from build123d import *

# Parameters (mm, degrees)
SKETCH_W             = 185.32
SKETCH_H             = 240.5
PAD_DEPTH            = 30
SKETCH003_W          = 145.32
SKETCH003_H          = 200.5
POCKET_DEPTH         = 23.6
SKETCH004_W          = 80.32
SKETCH004_H          = 135.5
POCKET001_DEPTH      = 6.4
POCKET002_DEPTH      = 3
SKETCH006_W          = 14
SKETCH006_H          = 3
POCKET003_DEPTH      = 30
POCKET004_DEPTH      = 1.5
SKETCH008_W          = 12
SKETCH008_H          = 2.4244
POCKET005_DEPTH      = 30
SKETCH009_W          = 87.32
SKETCH009_H          = 142.5
PAD001_DEPTH         = 4
SKETCH010_W          = 76.32
SKETCH010_H          = 131.5
POCKET006_DEPTH      = 0.001
POCKET006_DEPTH_BACK = -30.001
CHAMFER_SIZE         = 10
CHAMFER001_SIZE      = 5
CHAMFER002_SIZE      = 3


with BuildPart() as part:
    # Sketch → Pad (new body)
    with BuildSketch(Plane.XY):
        Rectangle(SKETCH_W, SKETCH_H)
    extrude(amount=PAD_DEPTH)

    # Sketch003 → Pocket (cut)
    with BuildSketch(Plane.XY.offset(30)):
        Rectangle(SKETCH003_W, SKETCH003_H)
    extrude(amount=-POCKET_DEPTH, mode=Mode.SUBTRACT)

    # Sketch004 → Pocket001 (cut)
    with BuildSketch(Plane.XY.offset(6.4)):
        Rectangle(SKETCH004_W, SKETCH004_H)
    extrude(amount=-POCKET001_DEPTH, mode=Mode.SUBTRACT)

    # Sketch005 → Pocket002 (cut)
    with BuildSketch(Plane.XY):
        with BuildLine():
            ThreePointArc((-85.97, 0), (-82.985, -2.985), (-80, 0))
            Line((-80, 0), (-80, 18.025988))
            ThreePointArc((-80, 18.025988), (-82.985, 27.495), (-85.97, 18.025988))
            Line((-85.97, 18.025988), (-85.97, 0))
        make_face()
    extrude(amount=POCKET002_DEPTH, mode=Mode.SUBTRACT)

    # Sketch006 → Pocket003 (cut, symmetric)
    with BuildSketch(Plane.XZ):
        with Locations((-83, 4.48)):
            Rectangle(SKETCH006_W, SKETCH006_H)
    extrude(amount=POCKET003_DEPTH, both=True, mode=Mode.SUBTRACT)

    # Sketch007 → Pocket004 (cut, symmetric)
    with BuildSketch(Plane.XY):
        with BuildLine():
            ThreePointArc((0, 110.985), (-2.985, 108), (0, 105.015))
            Line((0, 105.015), (18.705988, 105.015))
            ThreePointArc((18.705988, 105.015), (28.175, 108), (18.705988, 110.985))
            Line((18.705988, 110.985), (0, 110.985))
        make_face()
    extrude(amount=POCKET004_DEPTH, both=True, mode=Mode.SUBTRACT)

    # Sketch008 → Pocket005 (cut, symmetric)
    with BuildSketch(Plane.YZ):
        with Locations((108, 2.7105)):
            Rectangle(SKETCH008_W, SKETCH008_H)
    extrude(amount=POCKET005_DEPTH, both=True, mode=Mode.SUBTRACT)

    # Sketch009 → Pad001 (join)
    with BuildSketch(Plane.XY.offset(6.4)):
        Rectangle(SKETCH009_W, SKETCH009_H)
    extrude(amount=PAD001_DEPTH)

    # Sketch010 → Pocket006 (cut, two sides)
    with BuildSketch(Plane.XY) as pocket006_sk:
        Rectangle(SKETCH010_W, SKETCH010_H)
    extrude(amount=-POCKET006_DEPTH, mode=Mode.SUBTRACT)
    extrude(pocket006_sk.sketch, amount=-POCKET006_DEPTH_BACK, mode=Mode.SUBTRACT)

    # Chamfer
    chamfer_edges = [part.edges().sort_by_distance(p)[0] for p in [
        (-72.66, 0, 30),
        (0, 100.25, 30),
        (72.66, 0, 30),
        (0, -100.25, 30),
    ]]
    chamfer(chamfer_edges, length=CHAMFER_SIZE)

    # Chamfer001
    chamfer001_edges = [part.edges().sort_by_distance(p)[0] for p in [
        (0, 120.25, 30),
        (-92.66, 0, 30),
        (0, -120.25, 30),
        (92.66, 0, 30),
    ]]
    chamfer(chamfer001_edges, length=CHAMFER001_SIZE)

    # Chamfer002
    chamfer002_edges = [part.edges().sort_by_distance(p)[0] for p in [
        (-43.66, 0, 10.4),
        (0, -71.25, 10.4),
        (43.66, 0, 10.4),
        (0, 71.25, 10.4),
    ]]
    chamfer(chamfer002_edges, length=CHAMFER002_SIZE)


solid = part.part
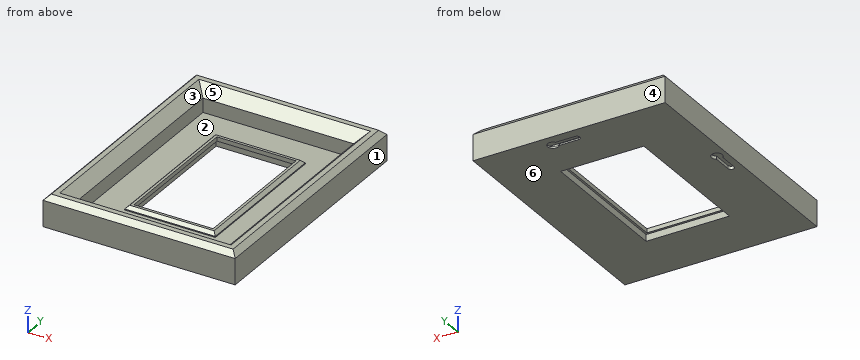
Part model, mm, in its own coordinate system. Face numbers are marked on the shaded views. A direction names the side the tool comes from. Coordinates: 2 decimals unless noted, no trailing zeros. Order: outer loops, then holes, each group sorted by start corner. A loop starts at its lowest first (then second) coordinate and runs counter-clockwise, first axis right, second up. Notation, with made-up numbers: (85.25, 54.5) - (89.25, 54.5) arc R8 ccw to (89.25, 65.5) - close; hole circle Ø5 at (16.25, 66). An arc over 180 degrees is marked (long way). Use CSV: the item, a comma, the result in double quotes.
Item 1: Drop a flat-ended pin along its axis: P1, Ø10, axis at x = -26.5, y = -70.5, coming from the +Z side. Give the stop position or say it passes through.
Solved:
P1,"stops at z = 10.4"
Item 2: Probe probe 1 along Y at (x, z) = (22.97, 0.95) (3 decimals); probe 2 along Y at (x, z) = (-23, 18); probe 3 along X at (y, z) = (83, 18). List the from-to ranges inside material, lowest first.
Solved:
probe 1,"y = -120.25 to -67.75, 67.75 to 102.795, 113.205 to 120.25"
probe 2,"y = -120.25 to -100.25, 100.25 to 120.25"
probe 3,"x = -92.66 to -72.66, 72.66 to 92.66"
Item 3: Mould opens along X. For the marked faces 1, 2, 3 and 4 say: +X half, -X half, draft (parallel to the pull), parting line (faces both ways), or undercut.
Solved:
face 1,"+X half"
face 2,"undercut"
face 3,"undercut"
face 4,"draft"
Item 4: 3-axis set-ups, long thin cutter, end or side, ignore diameter. For the marked faces 5 and 6: which of +Z, -Z, +X, -X, +Y, -Y reach the whole face in a straight line?
Solved:
face 5,"+Z"
face 6,"-Z, +X, -X, +Y, -Y"
Item 5: Saw through at B-B on x = -11.5. Give the number of separate pieces and of enclosed holes in the cut face, and give its area (3 significant figures).
Solved:
separate pieces,"2"
enclosed holes,"1"
area,"1,500 mm²"
Item 6: Saw through at D-D on y = -45.5. Give the cut face in (x, z).
Solved:
outline,"(-92.66, 0) - (-40.16, 0) - (-40.16, 6.4) - (-38.16, 6.4) - (-38.16, 10.4) - (-40.66, 10.4) - (-43.66, 7.4) - (-43.66, 6.4) - (-72.66, 6.4) - (-72.66, 20) - (-82.66, 30) - (-87.66, 30) - (-92.66, 25) - close; (38.16, 6.4) - (40.16, 6.4) - (40.16, 0) - (92.66, 0) - (92.66, 25) - (87.66, 30) - (82.66, 30) - (72.66, 20) - (72.66, 6.4) - (43.66, 6.4) - (43.66, 7.4) - (40.66, 10.4) - (38.16, 10.4) - close"
